Check sheet for the modelled part. Datum: model origin and axes. Units: mm. A direction names the side the tool comes from. Round coordinates to 2 decimals unless told otherwise and drop trailing zeros. Write each loop counter-clockwise with the first axis right and the second up, starting at its lowest first coordinate (ties: lowest second). Pieces come first, ordered by that corner, then holes. Notation, with made-up numbers: (-27.75, 79) -> (7.25, 79) arc R18 ccw to (7.25, 112) -> close; hole circle Ø1 at (22, 45.5). An arc over 180 degrees is marked (long way). One line per item, written item: value.
from build123d import *

# Parameters (mm, degrees)
F1_DEPTH = 8
F2_R     = 7.8
F2_R_2   = 6.8
F3_DEPTH = 7


with BuildPart() as f1:
    # F0 (on Front) → F1 (new body)
    with BuildSketch(Plane.XZ):
        with BuildLine():
            Line((20.9, 0), (4, 0))
            ThreePointArc((4, 0), (1.171573, -1.171573), (0, -4))
            Line((0, -4), (0, -45.9))
            ThreePointArc((0, -45.9), (1.171573, -48.728427), (4, -49.9))
            Line((4, -49.9), (20.9, -49.9))
            ThreePointArc((20.9, -49.9), (23.728427, -48.728427), (24.9, -45.9))
            Line((24.9, -45.9), (24.9, -4))
            ThreePointArc((24.9, -4), (23.728427, -1.171573), (20.9, 0))
        make_face()
    extrude(amount=F1_DEPTH)

    # F2 (on face) → F3 (cut)
    with BuildSketch(Plane.XZ.offset(8)):
        with Locations((9, -9)):
            Circle(F2_R)
        with Locations((15.9, -24)):
            Circle(F2_R_2)
        with Locations((9, -39)):
            Circle(F2_R)
    extrude(amount=-F3_DEPTH, mode=Mode.SUBTRACT)


solid = f1.part
Item 1: Release check for a two-part mould opening along X. For faces 3 (the cylindrical face through (23.697, -3.944, -48.759)), 4 (the flat face through (13, -4, 0)), 5 (the cylindrical face through (1.141, -3.944, -48.697)), 6 (the flat face through (9, -1, -39)) record: pulls with the +X half, pulls with the -X half, needs draft (parallel to the pull), parting line crosses it, or undercut.
Result set:
face 3: pulls with the +X half
face 4: needs draft
face 5: pulls with the -X half
face 6: undercut
Item 2: Sectioned sample at B-B (z = -24). Enter the section's corners in (x, y).
Result set:
outline: (0, -8) -> (9.1, -8) -> (9.1, -1) -> (22.7, -1) -> (22.7, -8) -> (24.9, -8) -> (24.9, 0) -> (0, 0) -> close
Item 3: Tool access check on faces 1 (the cylindrical face through (14.43, -4.55, -30.64)), 2 (the flat face through (12, -8, -30)). Record the directions out of +Z, -Z, +X, -X, +Y, -Y that give a thin tool (end or side, any length) a straight path to the whole face; none if there is none.
Result set:
face 1: -Y
face 2: +Z, -Z, +X, -X, -Y
Item 4: Material ranges on line 1 along Z through (x, y) = (9, -3.75); line 2 along Z through (x, y) = (10.5, -1.75); line 3 along Z through (x, y) = (15.9, -5), recorded low to high.
Result set:
line 1: -49.9 to -46.8, -31.2 to -16.8, -1.2 to 0
line 2: -49.9 to -46.65, -31.35 to -28.13, -19.87 to -16.65, -1.35 to 0
line 3: -49.9 to -42.64, -35.36 to -30.8, -17.2 to -12.64, -5.36 to 0
Item 5: Sectioned sample at C-C (x = 2). Enter the section's corners in (y, z).
Result set:
outline: (-8, -49.36) -> (0, -49.36) -> (0, -0.54) -> (-8, -0.54) -> (-8, -5.56) -> (-1, -5.56) -> (-1, -12.44) -> (-8, -12.44) -> (-8, -35.56) -> (-1, -35.56) -> (-1, -42.44) -> (-8, -42.44) -> close
Item 6: Depth check by flat-ended pin: pin 1 (8 mm diameter, centred on x = 12, z = -37, fed in from -Y). Enter the tip coordinate at first touch or a pass-through.
Result set:
pin 1: y = -1
Item 7: Sectioned sample at D-D (z = -42). Enter the section's corners in (x, y).
Result set:
outline: (0, -8) -> (1.8, -8) -> (1.8, -1) -> (16.2, -1) -> (16.2, -8) -> (24.9, -8) -> (24.9, 0) -> (0, 0) -> close
Item 8: Sectioned sample at A-A (y = -1.75). Enter the section's corners in (x, z).
Result set:
outline: (0, -45.9) arc R4 ccw to (4, -49.9) -> (20.9, -49.9) arc R4 ccw to (24.9, -45.9) -> (24.9, -4) arc R4 ccw to (20.9, 0) -> (4, 0) arc R4 ccw to (0, -4) -> close; hole circle Ø15.6 at (9, -39); hole circle Ø15.6 at (9, -9); hole circle Ø13.6 at (15.9, -24)
